Autodesk Inventor part; units mm, degrees
ref_plane "YZ Plane" through (0, 0, 0) normal (1, 0, 0) x (0, 1, 0)
ref_plane "XZ Plane" through (0, 0, 0) normal (0, 1, 0) x (-1, 0, 0)
ref_plane "XY Plane" through (0, 0, 0) normal (0, 0, 1) x (1, 0, 0)
sketch "Sketch1" plane through (0, 0, 0) normal (0, 1, 0) x (-1, 0, 0)
  line L0 (0, 0) -> (6, 0)
  line L1 (6, 0) -> (6, -17)
  line L2 (6, -17) -> (5.5, -17)
  line L3 (5.5, -17) -> (5.5, -17.7)
  line L4 (0, -19.7) -> (0, 0)
  line L5 (5.5, -17.7) -> (6, -17.7)
  line L6 (6, -17.7) -> (6, -18.7)
  line L7 (0, -19.7) -> (5, -19.7)
  line L8 (6, -18.7) -> (5, -19.7)
  line L9 (6, 0) -> (6, 17)
  line L10 (6, 17) -> (5.5, 17)
  line L11 (5.5, 17) -> (5.5, 17.7)
  line L12 (0, 19.7) -> (0, 0)
  line L13 (5.5, 17.7) -> (6, 17.7)
  line L14 (6, 17.7) -> (6, 18.7)
  line L15 (0, 19.7) -> (5, 19.7)
  line L16 (6, 18.7) -> (5, 19.7)
  point P0 (6, -19.7)
  dimension "d0" = 6
  dimension "d1" = 17
  dimension "d2" = 0.7
  dimension "d3" = 0.5
  dimension "d7" = 2
  dimension "d8" = 1
  dimension "d9" = 1
revolve "Revolution1" add sketch "Sketch1" angle 360 about axis through (0, 0, 19.7) along (0, 0, -1)
properties part number "Pin til stang"
Design review of the part built by this model. Coordinates are the model's own, in mm. A direction names the side the tool comes from. Coordinates: 2 decimals unless noted, no trailing zeros. Write each loop counter-clockwise with the first axis right and the second up, starting at its lowest first coordinate (ties: lowest second). Pieces come first, ordered by that corner, then holes. Notation, with made-up numbers: (-14, 9.5) -> (14, 9.5) arc R14 cw to (14, 27.5) -> close; hole circle Ø8 at (-3.75, -13.5). An arc over 180 degrees is marked (long way). Write each question's results on one line, items separated by ' | '. Start each with the question number.
(1) For line 1 along Z through (x, y) = (3.5, 4.5); line 2 along X through (y, z) = (-1, -11); line 3 along X through (y, z) = (-1.75, 16), list the stretches that pass through material, from the lowest coordinate up. Write a range as from..to.
(2) The part is to be moulded in two halves that separate along Z. For faces 3 (the face through (-3, -5, -17.7)), 4 (the face through (1.19, -5.37, -17.35)), 5 (the face through (0, 0, 19.7)), 6 (the face through (6, 0, 18)), say which applies: pulls with the +Z half, pulls with the -Z half, needs draft (parallel to the pull), parting line crosses it, or undercut.
(3) Tool access review of faces 1 (the face through (0, 0, -19.7)), 2 (the face through (-3, -5, -17)): name each direction out of +Z, -Z, +X, -X, +Y, -Y from which nothing blocks a thin tool from reaching the whole face with its end or side.
(4) Take a section at A-A on z = 7. Write out the cut boundary in (x, y), and give its area (3 significant figures).
(5) Clearance check with flat-ended pins moving along their axes: P1, Ø3, axis at y = -4, z = -0.5, coming from the +X side; P2, Ø1, axis at y = 1, z = 15, coming from the +X side. State where each tip first meets the part, or that it passes through.
Results found:
1) line 1: z = -19..-17.7, -17..17, 17.7..19 | line 2: x = -5.92..5.92 | line 3: x = -5.74..5.74
2) face 3: undercut | face 4: undercut | face 5: pulls with the +Z half | face 6: needs draft
3) face 1: -Z, +X, -X, +Y, -Y | face 2: none
4) outline: circle Ø12 at (0, 0) | area: 113 mm2
5) P1: stops at x = 5.45 | P2: stops at x = 5.98
